Geometry: final body of the model. Coordinates: model frame, mm. Face numbers are marked on the shaded views. A direction names the side the tool comes from. Give positions to 0.01 mm unless a question says otherwise; leave off trailing zeros. Loops run counter-clockwise (first coordinate to the right, second up) from the corner with the lowest first, then second, coordinate; pieces in that order, holes last.
```python
from build123d import *

# Parameters (mm, degrees)
REVOLUTION_ANGLE = -90
POCKET_DEPTH     = 3
PAD_DEPTH        = 102
PAD001_DEPTH     = 102
PAD002_DEPTH     = 102
SKETCH005_R      = 6
POCKET001_DEPTH  = 3
PAD003_DEPTH     = 80
PAD004_DEPTH     = 80


with BuildPart() as part:
    # Sketch → Revolution (revolve)
    with BuildSketch(Plane.XZ):
        Polygon((0, 0), (71, 0), (71, 5), (69, 5), (69, 3), (65, 3), (65, 105), (62, 105), (62, 3), (0, 3), align=None)
    revolve(axis=Axis((0, 0, 0), (0, 0, 1)), revolution_arc=REVOLUTION_ANGLE)

    # Sketch001 (on Face9 of Revolution) → Pocket (cut)
    with BuildSketch(Plane(origin=(0, 0, 3), x_dir=(-1, 0, 0), z_dir=(0, 0, 1))):
        Polygon((0, 0), (-30, 0), (0, 30), align=None)
    extrude(amount=-POCKET_DEPTH, mode=Mode.SUBTRACT)

    # Sketch002 (on Face7 of Pocket) → Pad (join)
    with BuildSketch(Plane(origin=(0, 0, 3), x_dir=(-1, 0, 0), z_dir=(0, 0, 1))):
        Polygon((0, 71), (0, 30), (-30, 0), (-71, 0), (-71, -3), (-28.7574, -3), (3, 28.7574), (3, 71), align=None)
    extrude(amount=PAD_DEPTH)

    # Sketch003 (on Face24 of Pad) → Pad001 (join)
    with BuildSketch(Plane(origin=(0, 0, 3), x_dir=(-1, 0, 0), z_dir=(0, 0, 1))):
        Polygon((0, 71), (0, 69), (-3.090822, 68.761632), (-3.090822, 70.761632), align=None)
    extrude(amount=PAD001_DEPTH)

    # Sketch004 (on Face28 of Pad001) → Pad002 (join)
    with BuildSketch(Plane(origin=(0, 0, 3), x_dir=(-1, 0, 0), z_dir=(0, 0, 1))):
        Polygon((-71, 0), (-69, 0), (-68.761632, 3.090822), (-70.761632, 3.090822), align=None)
    extrude(amount=PAD002_DEPTH)

    # Sketch005 (on Face18 of Pad002) → Pocket001 (cut)
    with BuildSketch(Plane(origin=(12.8787, -12.8787, 0), x_dir=(0.707107, 0.707107, 0), z_dir=(-0.707107, 0.707107, 0))):
        with Locations((0, -15)):
            Circle(SKETCH005_R)
    extrude(amount=-POCKET001_DEPTH, mode=Mode.SUBTRACT)

    # Sketch006 (on Face33 of Pocket001) → Pad003 (join)
    with BuildSketch(Plane(origin=(0, 0, 3), x_dir=(-1, 0, 0), z_dir=(0, 0, 1))):
        Polygon((-23.770153, 52.052386), (-18.11127, 57.70721), (-15.001117, 54.594824), (-20.66, 48.94), (-21.508224, 49.788833), (-17.264061, 54.029951), (-18.677767, 55.444672), (-22.92193, 51.203553), align=None)
        Polygon((-57.711085, 18.111455), (-52.053894, 23.767973), (-51.205416, 22.919394), (-55.448309, 18.677006), (-54.03418, 17.262708), (-49.791287, 21.505096), (-48.942809, 20.656518), (-54.6, 15), align=None)
    extrude(amount=PAD003_DEPTH)

    # Sketch006 (on Face33 of Pocket001) → Pad004 (join)
    with BuildSketch(Plane(origin=(0, 0, 3), x_dir=(-1, 0, 0), z_dir=(0, 0, 1))):
        Polygon((-23.770153, 52.052386), (-18.11127, 57.70721), (-15.001117, 54.594824), (-20.66, 48.94), (-21.508224, 49.788833), (-17.264061, 54.029951), (-18.677767, 55.444672), (-22.92193, 51.203553), align=None)
        Polygon((-57.711085, 18.111455), (-52.053894, 23.767973), (-51.205416, 22.919394), (-55.448309, 18.677006), (-54.03418, 17.262708), (-49.791287, 21.505096), (-48.942809, 20.656518), (-54.6, 15), align=None)
    extrude(amount=PAD004_DEPTH)


solid = part.part
```
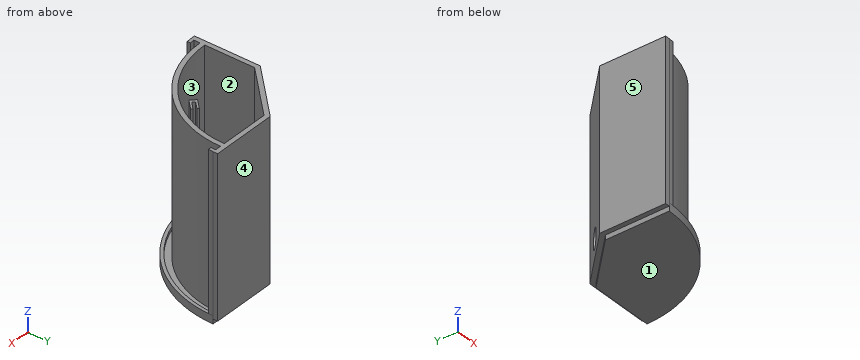
Q1. Material intervals for probe 1 along X at (y, z) = (-21, 11); probe 2 along X at (y, z) = (-17, 53); probe 3 along Y at (x, z) = (1, 24), sorted ascending.
Q2. Section query D-D, the plane z = 93. Return loops of the section in (x, y), and give its area (3 significant figures).
Q3. Mould query, pull axis X, two halves, no side actions, for the marked faces 3, 4 and 5. Classes: +X half, -X half, draft (parallel to the pull), parting line (faces both ways), or undercut.
Q4. Section query A-A, the plane z = 77.5. State how many separate pieces and enclosed holes the cut face has, and give its area (3 significant figures).
Q5. Reachability of the marked faces 1 and 2 from +Z, -Z, +X, -X, +Y, -Y: full face, straight path, thin tool, end or side. Return the list, or none.
Q6. Pin query (flat end, axial travel): pin 1 Ø6 at (x, y) = (7, -20) entering from -Z; pin 2 Ø4.5 at (x, y) = (19, -53) entering from +Z; pin 3 Ø0.6 at (y, z) = (-70, 49.5) entering from +X; pin 4 Ø6 at (y, z) = (-8.5, 59.5) entering from -X. Return the tip coordinate at first contact, or that it passes through.
Resolved:
1. probe 1: x = 4.76 to 9, 49.29 to 50.3, 53.13 to 54.82, 58.34 to 61.51
1. probe 2: x = 8.76 to 13, 52.6 to 56.6, 59.62 to 62.74
1. probe 3: y = -70.92 to -68.92, -64.99 to -61.99, -29 to -24.76
2. outline: (-3, -71) - (0, -71) - (3.09, -70.76) - (3.09, -68.76) - (0, -69) - (0, -65) arc R65 ccw to (65, 0) - (69, 0) - (68.76, -3.09) - (70.76, -3.09) - (71, 0) - (71, 3) - (28.76, 3) - (-3, -28.76) - close; hole (0, -62) arc R62 ccw to (62, 0) - (30, 0) - (0, -30) - close
2. area: 692 mm2
3. face 3: undercut
3. face 4: draft
3. face 5: -X half
4. separate pieces: 3
4. enclosed holes: 1
4. area: 739 mm2
5. face 1: -Z, +X, -X, +Y, -Y
5. face 2: +Z
6. pin 1: stops at z = 0
6. pin 2: stops at z = 83
6. pin 3: stops at x = 3.09
6. pin 4: stops at x = 14.26
